Autodesk Inventor part; units mm, degrees
ref_plane "YZ Plane" through (0, 0, 0) normal (1, 0, 0) x (0, 1, 0)
ref_plane "XZ Plane" through (0, 0, 0) normal (0, 1, 0) x (-1, 0, 0)
ref_plane "XY Plane" through (0, 0, 0) normal (0, 0, 1) x (1, 0, 0)
sketch "Sketch1" plane through (0, 0, 0) normal (0, 0, 1) x (1, 0, 0)
  circle A0 centre (0, 0) radius 3
  dimension "d0" = 6
extrude "Extrusion1" add sketch "Sketch1" along normal blind 101.6
chamfer "Chamfer1" distance 0.254 distance2 0.762 1 edges at (-3, 0, 0) measured on face at (-0.5351, 1.0949, 0)
chamfer "Chamfer2" distance 0.254 distance2 0.762 1 edges at (-3, 0, 101.6) measured on face at (-0.5351, 1.0949, 101.6)
sketch "Sketch2" plane through (0, 0, 0) normal (0, 0, -1) x (-1, 0, 0)
  circle A0 centre (0, 0) radius 2.746
sketch "Sketch3" plane through (0, 0, 101.6) normal (0, 0, 1) x (1, 0, 0)
  circle A0 centre (0, 0) radius 2.746
hole "Hole1" at (0, 0, 0) direction (0, 0, 1) diameter 2.156 depth 5 tip angle 118
hole "Hole2" at (0, 0, 101.6) direction (0, 0, -1) diameter 2.156 depth 5 tip angle 118
properties part number "ER4_CageRod"
Input: part model. Units: mm. Frame: model coordinates. A direction names the side the tool comes from. Round coordinates to 2 decimals unless told otherwise and drop trailing zeros. One line per question, with ' | ' between items. Start each with the question number.
1) Contact query for flat-ended pins moving along their axis: P1, Ø1.5, axis at y = 1.5, z = 25, coming from the -X side; P2, Ø1.3, axis at x = 0, y = 0, coming from the +Z side. Output: stop coordinate, or through.
2) Ray query, probe 1 along Y at (x, z) = (0, 1.6); probe 2 along X at (y, z) = (-1.2, 65); probe 3 along X at (y, z) = (-0.15, 70.5). Return the intervals inside material, ascending.
3) Pull-direction query (X, two-part tool) for faces 1 (the cylindrical face through (-0.32, 1.03, 2.54)), 2 (the flat face through (1, -1, 101.6)), 3 (the cylindrical face through (-3, 0, 50)); classes: +X half, -X half, draft (parallel to the pull), parting line (faces both ways), or undercut.
4) Set-up query: faces 4 (the flat face through (1, -1, 0)), 5 (the cylindrical face through (-0.32, -1.03, 99.06)). Return all of +Z, -Z, +X, -X, +Y, -Y with unobstructed straight access to the full face (end or side cutting, diameter ignored); none if empty.
Worked out:
1) P1: stops at x = -2.9 | P2: stops at z = 96.34
2) probe 1: y = -3 to -1.08, 1.08 to 3 | probe 2: x = -2.75 to 2.75 | probe 3: x = -3 to 3
3) face 1: undercut | face 2: draft | face 3: parting line
4) face 4: -Z, +X, -X, +Y, -Y | face 5: +Z
